```python
from build123d import *

# Parameters (mm, degrees)
SKETCH1_R           = 7.5
BOSS_EXTRUDE1_DEPTH = 7.5
FILLET1_R           = 1
SKETCH2_R           = 4.5
BOSS_EXTRUDE2_DEPTH = 6
SKETCH3_W           = 5
SKETCH3_H           = 5
BOSS_EXTRUDE3_DEPTH = 3


with BuildPart() as part:
    # Sketch1 → Boss-Extrude1 (new body)
    with BuildSketch(Plane(origin=(0, 0, 0), x_dir=(1, 0, 0), z_dir=(0, 1, 0))):
        with Locations(Location((0, 0, 0), (0, 0, 270))):
            Circle(SKETCH1_R)
    extrude(amount=BOSS_EXTRUDE1_DEPTH)

    # Fillet1
    fillet1_edges = [part.edges().sort_by_distance(p)[0] for p in [
        (0, 7.5, -7.5),
    ]]
    fillet(fillet1_edges, radius=FILLET1_R)

    # Sketch2 → Boss-Extrude2 (add)
    with BuildSketch(Plane(origin=(0, 0, 0), x_dir=(-1, 0, 0), z_dir=(0, -1, 0))):
        with Locations(Location((0, 0, 0), (0, 0, 90))):
            Circle(SKETCH2_R)
    extrude(amount=BOSS_EXTRUDE2_DEPTH)

    # Sketch3 → Boss-Extrude3 (add)
    with BuildSketch(Plane(origin=(0, -6, 0), x_dir=(-1, 0, 0), z_dir=(0, -1, 0))):
        Rectangle(SKETCH3_W, SKETCH3_H)
    extrude(amount=BOSS_EXTRUDE3_DEPTH)


solid = part.part
```
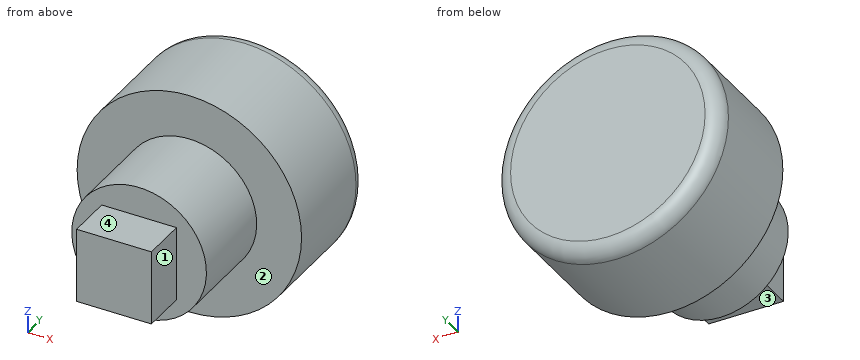
For this review, take the finished solid that the model builds, in its own axes (mm). Face numbers are marked on the shaded views. A direction names the side the tool comes from. Coordinates: 2 decimals unless noted, no trailing zeros. Loops run counter-clockwise (first coordinate to the right, second up) from the corner with the lowest first, then second, coordinate; pieces in that order, holes last.
1. Add section B-B, the plane x = 0. Give the boundary of the cut face in (y, z).
2. Add section C-C, the plane y = 3. Give the boundary of the cut face in (x, z), then the cut area to 3 significant figures.
3. Insertion check: P1, Ø3, axis at x = 5, y = 5, coming from the -Z side; P2, Ø1.5, axis at x = -4.5, y = -5, coming from the -Z side; P3, Ø1.5, axis at y = -4.5, z = -3.5, coming from the +X side; P4, Ø5, axis at x = 0, y = -1, coming from the +Z side. Each pin has a flat end and moves straight along its axis. Give the tip position at first contact, or say it passes through.
4. Add section A-A, the plane z = 0. Give the boundary of the cut face in (x, y).
5. For line 1 (X direction, y = 1.5, z = 0.25); line 2 (Z direction, x = 1.25, y = -8.5); line 3 (Y direction, x = 3.25, z = -1.75), list the stretches that pass through material, from the lowest coordinate up.
6. For the marked faces 1, 2, 3 and 4, list the 3-axis set-ups (+Z, -Z, +X, -X, +Y, -Y) from which the entire face can be reached by the end or side of a thin tool; tool diameter is ignored.
7. Add section D-D, the plane y = -5.5. Give the boundary of the cut face in (x, z), then the cut area to 3 significant figures.
Result:
1. outline: (-9, -2.5) - (-6, -2.5) - (-6, -4.5) - (0, -4.5) - (0, -7.5) - (6.5, -7.5) arc R1 ccw to (7.5, -6.5) - (7.5, 6.5) arc R1 ccw to (6.5, 7.5) - (0, 7.5) - (0, 4.5) - (-6, 4.5) - (-6, 2.5) - (-9, 2.5) - close
2. outline: circle Ø15 at (0, 0)
2. area: 177 mm2
3. P1: stops at z = -6.63
3. P2: stops at z = -2.49
3. P3: stops at x = 3.56
3. P4: stops at z = 7.5
4. outline: (-7.5, 0) - (-4.5, 0) - (-4.5, -6) - (-2.5, -6) - (-2.5, -9) - (2.5, -9) - (2.5, -6) - (4.5, -6) - (4.5, 0) - (7.5, 0) - (7.5, 6.5) arc R1 ccw to (6.5, 7.5) - (-6.5, 7.5) arc R1 ccw to (-7.5, 6.5) - close
5. line 1: x = -7.5 to 7.5
5. line 2: z = -2.5 to 2.5
5. line 3: y = -6 to 7.5
6. face 1: +Z, -Z, +X, -Y
6. face 2: -Y
6. face 3: -Z, +X, -X, -Y
6. face 4: +Z, +X, -X, -Y
7. outline: circle Ø9 at (0, 0)
7. area: 63.6 mm2
